Source: CAD feature listing. Evaluate the final solid. Frame: model axes, mm. A direction names the side the tool comes from. Give positions to 0.01 mm unless a question says otherwise; leave off trailing zeros. Write each loop counter-clockwise with the first axis right and the second up, starting at its lowest first coordinate (ties: lowest second). Pieces come first, ordered by that corner, then holes. Notation, with made-up numbers: M 20.25,-9.5 L 75.25,-9.5 A18 cw 75.25,-4.5 Z; hole C -18,86 d8. An arc over 180 degrees is marked long. Return JSON: item names as keys, results as strings.
Autodesk Inventor part; units mm, degrees
ref_plane "YZ Plane" through (0, 0, 0) normal (1, 0, 0) x (0, 1, 0)
ref_plane "XZ Plane" through (0, 0, 0) normal (0, 1, 0) x (-1, 0, 0)
ref_plane "XY Plane" through (0, 0, 0) normal (0, 0, 1) x (1, 0, 0)
sketch "Sketch1" plane through (0, 0, 0) normal (0, 0, 1) x (1, 0, 0)
  circle A0 centre (0, 0) radius 9.4742
  dimension "d0" = 18.9484
extrude "Extrusion1" add sketch "Sketch1" against normal blind 3.81
sketch "Sketch2" plane through (0, 0, 0) normal (0, 0, 1) x (1, 0, 0)
  circle A0 centre (0, 0) radius 4.5085
  dimension "d3" = 9.017
extrude "Extrusion2" add sketch "Sketch2" against normal blind 32.639
sketch "Sketch3" plane through (0, 0, 0) normal (0, 0, 1) x (1, 0, 0)
  circle A0 centre (0, 0) radius 3.4925
  dimension "d6" = 6.985
extrude "Extrusion3" add sketch "Sketch3" against normal blind 38.1
sketch "Sketch4" plane through (0, 0, 0) normal (0, 0, 1) x (1, 0, 0)
  circle A0 centre (0, 0) radius 2.413
  dimension "d9" = 4.826
extrude "Extrusion4" add sketch "Sketch4" against normal blind 54.61
sketch "Sketch6" plane through (0, 0, 0) normal (0, 0, 1) x (1, 0, 0)
  circle A0 centre (0, 0) radius 9.4742
hole "Hole1" at (0, 0, 0) direction (0, 0, -1) diameter 6.5278 depth 22.352
sketch "Sketch5" plane through (0, 0, 0) normal (0, 1, 0) x (-1, 0, 0)
  line L0 (-4.5085, -32.639) -> (4.5085, -32.639)
  line L1 (4.5085, -3.81) -> (-4.5085, -3.81)
  line L2 (-3.4925, -38.1) -> (3.4925, -38.1)
  line L3 (3.4925, -32.639) -> (-3.4925, -32.639)
  line L4 (-3.4925, -32.639) -> (-3.4925, -38.1)
  line L5 (-2.413, -38.1) -> (-2.413, -54.61)
  line L6 (3.4925, -32.639) -> (3.4925, -38.1)
  line L7 (4.5085, -3.81) -> (4.5085, -32.639)
  line L8 (-4.5085, -3.81) -> (-4.5085, -32.639)
  line L9 (9.4742, 0) -> (9.4742, -3.81)
  line L10 (-9.4742, -3.81) -> (9.4742, -3.81)
  line L11 (-9.4742, 0) -> (9.4742, 0)
  line L12 (-9.4742, 0) -> (-9.4742, -3.81)
  line L13 (2.413, -38.1) -> (2.413, -54.61)
  line L14 (-2.413, -54.61) -> (2.413, -54.61)
  line L15 (-3.4925, -32.639) -> (-3.4925, -34.036) construction
  line L16 (-3.4925, -38.1) -> (3.4925, -38.1)
  line L17 (-3.4925, -34.036) -> (-2.5273, -34.036)
  line L18 (-2.5273, -34.036) -> (-2.5273, -38.1)
  line L19 (-2.5273, -38.1) -> (-3.4925, -38.1)
  line L20 (-3.4925, -38.1) -> (-3.4925, -34.036)
  line L21 (3.4925, -34.036) -> (2.5273, -34.036)
  line L22 (2.5273, -34.036) -> (2.5273, -38.1)
  line L23 (2.5273, -38.1) -> (3.4925, -38.1)
  line L24 (3.4925, -38.1) -> (3.4925, -34.036)
  point P0 (0, 0)
  dimension "d12" = 1.397
  dimension "d13" = 0.9652
  dimension "d14" = 0.9652
extrude "Extrusion5" cut sketch "Sketch5" along normal through all both and the other way through all contours L17 L18 L2 L4 | L6 L2 L22 L21
sketch "Sketch7" plane through (0, 0, 0) normal (0, 1, 0) x (-1, 0, 0)
  line L0 (-9.4742, 0) -> (9.4742, 0)
  line L1 (9.4742, 0) -> (9.4742, -3.81)
  line L2 (4.5085, -3.81) -> (4.5085, -32.639)
  line L3 (3.2639, -22.352) -> (3.2639, 0)
  line L4 (-3.2639, -22.352) -> (-3.2639, 0)
  line L5 (3.2639, -22.352) -> (-3.2639, -22.352)
  line L6 (-4.5085, -3.81) -> (-4.5085, -32.639)
  line L7 (-9.4742, 0) -> (-9.4742, -3.81)
  line L8 (3.4925, -32.639) -> (3.4925, -34.036)
  line L9 (3.4925, -34.036) -> (2.5273, -34.036)
  line L10 (2.5273, -38.1) -> (2.5273, -34.036)
  line L11 (2.413, -38.1) -> (2.413, -54.61)
  line L12 (-2.413, -38.1) -> (-2.413, -54.61)
  line L13 (-2.5273, -34.036) -> (-2.5273, -38.1)
  line L14 (-3.4925, -32.639) -> (-3.4925, -34.036)
  line L15 (9.4742, 0) -> (9.4742, -10.668)
  line L16 (4.5085, -10.668) -> (-0.0127, -10.668)
  line L17 (-0.0127, -10.668) -> (-0.0127, -20.1168)
  line L18 (-0.0127, -20.1168) -> (4.5085, -20.1168)
  line L19 (4.5085, -20.1168) -> (4.5085, -10.668)
  point P0 (0, 0)
  dimension "d26" = 10.668
  dimension "d27" = 9.4488
  dimension "d42" = 4.5212
extrude "Extrusion6" cut sketch "Sketch7" along normal through all contours L16 L2 L18 L3 | L3 L18 L17 L16
sketch "Sketch9" plane through (0, 0, 0) normal (0, 0, 1) x (1, 0, 0)
  line L0 (0, 0) -> (-6.9342, 0)
  circle A0 centre (-6.9342, 0) radius 1.7399
  dimension "d35" = 6.9342
  dimension "d36" = 3.4798
extrude "Extrusion8" add sketch "Sketch9" along normal blind 4.826
sketch "Sketch10" plane through (-6.9342, 0, 4.826) normal (0, 0, 1) x (1, 0, 0)
  circle A0 centre (0, 0) radius 1.5875
  point P0 (6.9342, 0)
  dimension "d39" = 3.175
extrude "Extrusion9" add sketch "Sketch10" along normal blind 2.159
sketch "Sketch8" plane through (0, 0, 0) normal (0, 0, 1) x (1, 0, 0)
  circle A0 centre (0, 0) radius 9.4742
  line L0 (0, -9.4742) -> (0, -6.2992)
  line L1 (0, -6.2992) -> (-8.9758, -3.0323)
  line L2 (0, 9.4742) -> (0, 6.2992)
  line L3 (0, 6.2992) -> (-8.9758, 3.0323)
  dimension "d30" = 3.175
  dimension "d31" = 110
  dimension "d32" = 3.175
extrude "Extrusion7" cut sketch "Sketch8" against normal through all contours L2 L3 A0 | A0 L1 L0
thread "Thread1"
properties part number "CrankShaft"
1) Cut plane D-D, the plane y = 8. Return the cut outline in (x, z).
Numbers:
{"outline": "M 0,-3.81 L 5.08,-3.81 L 5.08,0 L 0,0 Z"}
2) Draft query along X for faces 1 (the face through (2.9, -1.5, -11.3)), 2 (the face through (9.47, -0.21, -1.88)), 3 (the face through (4, -4, -3.81)), 4 (the face through (0, 8, -2)). Return one class per face: released by +X, released by -X, zero draft, split by the parting line, or undercut.
Numbers:
{"face 1": "undercut", "face 2": "released by +X", "face 3": "zero draft", "face 4": "released by -X"}
3) Contact query for flat-ended pins moving along their axis: pin 1 Ø2 at (y, z) = (0, -36) entering from -X; pin 2 Ø1 at (x, z) = (1, -22) entering from -Y; pin 3 Ø2 at (y, z) = (0, -35) entering from +X; pin 4 Ø1.5 at (y, z) = (-4, -46) entering from -X. Output: stop coordinate, or through.
Numbers:
{"pin 1": "stops at x = -2.53", "pin 2": "stops at y = -4.48", "pin 3": "stops at x = 3.49", "pin 4": "passes through"}
4) Line query: line 1 (Z direction, x = -2.5, y = 2.75); line 2 (X direction, y = 0, z = -7). Output: solid intervals per line, ascending. Write a range as [from, to].
Numbers:
{"line 1": "z = [-32.64, -20.12], [-10.67, 0]", "line 2": "x = [-4.51, -3.26], [3.26, 4.51]"}
5) Cut plane A-A, the plane z = -44. Return the cut outline in (x, y), then the cut area to 3 significant figures.
Numbers:
{"outline": "C 0,0 d4.83", "area": "18.3 mm²"}
6) Cut plane C-C, the plane z = -6. Return the cut outline in (x, y), then the cut area to 3 significant figures.
Numbers:
{"outline": "C 0,0 d9.02; hole C 0,0 d6.53", "area": "30.4 mm²"}
7) Set-up query: faces 5 (the face through (-3, 2, -10.668)), 6 (the face through (0, -4, -32.639)), 7 (the face through (0, -8, -2)). Return all of +Z, -Z, +X, -X, +Y, -Y with unobstructed straight access to the full face (end or side cutting, diameter ignored); none if empty.
Numbers:
{"face 5": "-X, +Y", "face 6": "-Z", "face 7": "+Z, -Z, -X, -Y"}
8) Cut plane B-B, the plane x = 1.5. Return the cut outline in (y, z), then the cut area to 3 significant figures.
Numbers:
{"outline": "M -9.35,-3.81 L -4.25,-3.81 L -4.25,-32.64 L -3.15,-32.64 L -3.15,-38.1 L -1.89,-38.1 L -1.89,-54.61 L 1.89,-54.61 L 1.89,-38.1 L 3.15,-38.1 L 3.15,-32.64 L 4.25,-32.64 L 4.25,-3.81 L 9.35,-3.81 L 9.35,0 L 2.9,0 L 2.9,-22.35 L -2.9,-22.35 L -2.9,0 L -9.35,0 Z", "area": "284 mm²"}
